```python
from build123d import *

# Parameters (mm, degrees)
SKETCH1_W           = 135
SKETCH1_H           = 90
SKETCH1_R           = 10
SKETCH1_R_2         = 5
BOSS_EXTRUDE2_DEPTH = 30
SKETCH2_R           = 9.5
CUT_EXTRUDE2_DEPTH  = 20
SKETCH3_R           = 8
CUT_EXTRUDE3_DEPTH  = 10


with BuildPart() as part:
    # Sketch1 → Boss-Extrude2 (new body)
    with BuildSketch(Plane(origin=(0, 0, 0), x_dir=(1, 0, 0), z_dir=(0, 1, 0))):
        Rectangle(SKETCH1_W, SKETCH1_H)
        with Locations(Location((0, 22.5, 0), (0, 0, 270))):
            Circle(SKETCH1_R, mode=Mode.SUBTRACT)
        with Locations(Location((0, -22.5, 0), (0, 0, 270))):
            Circle(SKETCH1_R_2, mode=Mode.SUBTRACT)
        with Locations(Location((-45, -22.5, 0), (0, 0, 270))):
            Circle(SKETCH1_R_2, mode=Mode.SUBTRACT)
        with Locations(Location((45, -22.5, 0), (0, 0, 270))):
            Circle(SKETCH1_R_2, mode=Mode.SUBTRACT)
    extrude(amount=BOSS_EXTRUDE2_DEPTH)

    # Sketch2 → Cut-Extrude2 (cut)
    with BuildSketch(Plane(origin=(0, 30, 0), x_dir=(1, 0, 0), z_dir=(0, 1, 0))):
        with Locations(Location((-45, 22.5, 0), (0, 0, 270))):
            Circle(SKETCH2_R)
        with Locations(Location((45, 22.5, 0), (0, 0, 90))):
            Circle(SKETCH2_R)
    extrude(amount=-CUT_EXTRUDE2_DEPTH, mode=Mode.SUBTRACT)

    # Sketch3 → Cut-Extrude3 (cut)
    with BuildSketch(Plane.XZ):
        with Locations(Location((45, 22.5, 0), (0, 0, 270))):
            Circle(SKETCH3_R)
        with Locations(Location((0, 22.5, 0), (0, 0, 270))):
            Circle(SKETCH3_R)
        with Locations(Location((-45, 22.5, 0), (0, 0, 90))):
            Circle(SKETCH3_R)
    extrude(amount=-CUT_EXTRUDE3_DEPTH, mode=Mode.SUBTRACT)


solid = part.part
```
Work out the finished part from the listing and answer in its coordinate system (mm). A direction names the side the tool comes from. Give positions to 0.01 mm unless a question says otherwise; leave off trailing zeros. Write each loop counter-clockwise with the first axis right and the second up, starting at its lowest first coordinate (ties: lowest second). Pieces come first, ordered by that corner, then holes. Notation, with made-up numbers: (60.5, 23.25) - (111.5, 23.25) arc R29 ccw to (111.5, 62.25) - close; hole circle Ø6 at (-5, -17.5). An arc over 180 degrees is marked (long way). Use one line per item in the form item = value.
1. Determine the mould class of faces 4 (the face through (49, 10, 19)), 5 (the face through (-1, 30, -1)), 6 (the face through (-1, 15, 45)) for opening direction Z: released by +Z, released by -Z, zero draft, split by the parting line, or undercut.
Filled in:
face_4 = undercut
face_5 = zero draft
face_6 = released by +Z
2. A cutting plane is placed at C-C (y = 5.25). Write down the section's boundary in (x, z).
Filled in:
outline = (-67.5, -45) - (67.5, -45) - (67.5, 45) - (-67.5, 45) - close; hole circle Ø16 at (-45, 22.5); hole circle Ø20 at (0, -22.5); hole circle Ø16 at (0, 22.5); hole circle Ø16 at (45, 22.5)
3. A cutting plane is placed at A-A (z = -22.5). Write down the section's boundary in (x, y).
Filled in:
outline = (-67.5, 0) - (-10, 0) - (-10, 30) - (-35.5, 30) - (-35.5, 10) - (-54.5, 10) - (-54.5, 30) - (-67.5, 30) - close; (10, 0) - (67.5, 0) - (67.5, 30) - (54.5, 30) - (54.5, 10) - (35.5, 10) - (35.5, 30) - (10, 30) - close
4. A cutting plane is placed at B-B (x = 0). Write down the section's boundary in (y, z).
Filled in:
outline = (0, -45) - (30, -45) - (30, -32.5) - (0, -32.5) - close; (0, -12.5) - (30, -12.5) - (30, 17.5) - (10, 17.5) - (10, 14.5) - (0, 14.5) - close; (0, 30.5) - (10, 30.5) - (10, 27.5) - (30, 27.5) - (30, 45) - (0, 45) - close
5. Consider L1, parallel to X at y = 24.75, z = -22.5; L2, parallel to X at y = 6, z = 22.5; L3, parallel to Z at x = 1, y = 13.75. Determine where each line is inside the solid, lowest interval first.
Filled in:
L1 = -67.5 to -54.5, -35.5 to -10, 10 to 35.5, 54.5 to 67.5
L2 = -67.5 to -53, -37 to -8, 8 to 37, 53 to 67.5
L3 = -45 to -32.45, -12.55 to 17.6, 27.4 to 45
6. For faces 1 (the face through (4, 10, 19)), 2 (the face through (3, 14.79, -12.96)), 3 (the face through (36.99, 20.14, -27.61)), determine the directions among +Z, -Z, +X, -X, +Y, -Y from which every point of the face is accessible in a straight line to the end or side of a thin tool.
Filled in:
face_1 = -Y
face_2 = +Y, -Y
face_3 = +Y
7. A cutting plane is placed at D-D (z = 22.5). Write down the section's boundary in (x, y).
Filled in:
outline = (-67.5, 0) - (-53, 0) - (-53, 10) - (-50, 10) - (-50, 30) - (-67.5, 30) - close; (-40, 10) - (-37, 10) - (-37, 0) - (-8, 0) - (-8, 10) - (-5, 10) - (-5, 30) - (-40, 30) - close; (5, 10) - (8, 10) - (8, 0) - (37, 0) - (37, 10) - (40, 10) - (40, 30) - (5, 30) - close; (50, 10) - (53, 10) - (53, 0) - (67.5, 0) - (67.5, 30) - (50, 30) - close
8. This flat-tipped pin is pushed along its axis until it touches: pin 1 Ø13 at (x, z) = (-45, 22.5) entering from -Y. Where does it stop, or does it pass through?
Filled in:
pin_1 = 10
